The model under review builds one solid part; all positions refer to its coordinate system, in mm. Coordinates: 2 decimals unless noted, no trailing zeros. Order: outer loops, then holes, each group sorted by start corner. A loop starts at its lowest first (then second) coordinate and runs counter-clockwise, first axis right, second up. Notation, with made-up numbers: (21, 21.25) -> (54, 21.25) arc R28 cw to (54, 53.25) -> close; hole circle Ø1 at (28.25, 72). An arc over 180 degrees is marked (long way). Use one line per item in the form item = value. Start each with the question number.
(1) Wall thickness on line 1 along Z through (x, y) = (1.55, 0.1); line 2 along Z through (x, y) = (1.8, -0.15); line 3 along X through (y, z) = (-0.1, 17.75): over which ranges is each line inside the solid? List them lowest first.
(2) Mouldability with a two-part tool opening along Z and no side actions: class faces 1 (the cylindrical face through (-1.5, 0.07, 13.56)), 2 (the flat face through (0, 0, -1)), 3 (the cylindrical face through (-0.434, -1.952, 27.746)) as +Z half, -Z half, draft (parallel to the pull), parting line (faces both ways), or undercut.
(3) Take a section at C-C (z = 25.5). State the section outline as (x, y) points.
(4) Insertion check: pin 1 Ø1.5 at (x, z) = (-0.5, 2.5) entering from +Y; pin 2 Ø2 at (x, z) = (-1, 6) entering from -Y. Each pin has a flat end and moves straight along its axis. Give the tip position at first contact, or say it passes through.
(5) Take a section at A-A (y = 0). State the section outline as (x, z) points, then the cut area to 3 significant figures.
```python
from build123d import *

# Parameters (mm, degrees)
SKETCH1_R           = 1.5
BOSS_EXTRUDE1_DEPTH = 27.5
SKETCH2_R           = 2
BOSS_EXTRUDE2_DEPTH = 1
SKETCH3_R           = 2
BOSS_EXTRUDE3_DEPTH = 1
FILLET1_R           = 0.5


with BuildPart() as part:
    # Sketch1 → Boss-Extrude1 (new body)
    with BuildSketch(Plane.XY):
        Circle(SKETCH1_R)
    extrude(amount=BOSS_EXTRUDE1_DEPTH)

    # Sketch2 → Boss-Extrude2 (add)
    with BuildSketch(Plane(origin=(0, 0, 0), x_dir=(-1, 0, 0), z_dir=(0, 0, -1))):
        Circle(SKETCH2_R)
    extrude(amount=BOSS_EXTRUDE2_DEPTH)

    # Sketch3 → Boss-Extrude3 (add)
    with BuildSketch(Plane.XY.offset(27.5)):
        Circle(SKETCH3_R)
    extrude(amount=BOSS_EXTRUDE3_DEPTH)

    # Fillet1
    fillet1_edges = [part.edges().sort_by_distance(p)[0] for p in [
        (-2, 0, 28.5),
        (2, 0, -1),
    ]]
    fillet(fillet1_edges, radius=FILLET1_R)


solid = part.part
```
Findings:
q1.line_1 = -1 to 0, 27.5 to 28.5
q1.line_2 = -0.9 to 0, 27.5 to 28.4
q1.line_3 = -1.5 to 1.5
q2.face_1 = undercut
q2.face_2 = -Z half
q2.face_3 = draft
q3.outline = circle Ø3 at (0, 0)
q4.pin_1 = 1.5
q4.pin_2 = -1.5
q5.outline = (-2, -0.5) arc R0.5 ccw to (-1.5, -1) -> (1.5, -1) arc R0.5 ccw to (2, -0.5) -> (2, 0) -> (1.5, 0) -> (1.5, 27.5) -> (2, 27.5) -> (2, 28) arc R0.5 ccw to (1.5, 28.5) -> (-1.5, 28.5) arc R0.5 ccw to (-2, 28) -> (-2, 27.5) -> (-1.5, 27.5) -> (-1.5, 0) -> (-2, 0) -> close
q5.area = 90.3 mm²
